from build123d import *

# Parameters (mm, degrees)
ESTRUSIONE_ESTRUSIONE5_DEPTH = 34
ESTRUSIONE_ESTRUSIONE6_DEPTH = 32
SCHIZZO9_R                   = 14.5
ESTRUSIONE_ESTRUSIONE7_DEPTH = 8
SCHIZZO10_R                  = 8
TAGLIO_ESTRUSIONE1_DEPTH     = 104.947101932
SCHIZZO11_R                  = 3
TAGLIO_ESTRUSIONE2_DEPTH     = 98.923439482
NERVATURA1_START             = -3
NERVATURA1_DEPTH             = 6
NERVATURA11_START            = -3
NERVATURA11_DEPTH            = 6


with BuildPart() as part:
    # Schizzo7 → Estrusione-Estrusione5 (new, symmetric)
    with BuildSketch(Plane(origin=(0, 0, 0), x_dir=(1, 0, 0), z_dir=(0, 1, 0))):
        Polygon((-57, 20), (-57, -20), (-47, -20), (-47, 10), (57, 10), (57, 50), (47, 50), (47, 20), align=None)
    extrude(amount=ESTRUSIONE_ESTRUSIONE5_DEPTH, both=True)

    # Schizzo8 → Estrusione-Estrusione6 (add)
    with BuildSketch(Plane.XY.offset(-10)):
        with BuildLine():
            Line((-27.5, 5.656854249), (-4.833333333, 13.670731103))
            ThreePointArc((-4.833333333, 13.670731103), (0, 14.5), (4.833333333, 13.670731103))
            Line((4.833333333, 13.670731103), (27.5, 5.656854249))
            ThreePointArc((27.5, 5.656854249), (31.5, 0), (27.5, -5.656854249))
            Line((27.5, -5.656854249), (4.833333333, -13.670731103))
            ThreePointArc((4.833333333, -13.670731103), (0, -14.5), (-4.833333333, -13.670731103))
            Line((-4.833333333, -13.670731103), (-27.5, -5.656854249))
            ThreePointArc((-27.5, -5.656854249), (-31.5, 0), (-27.5, 5.656854249))
        make_face()
    extrude(amount=ESTRUSIONE_ESTRUSIONE6_DEPTH)

    # Schizzo9 → Estrusione-Estrusione7 (add)
    with BuildSketch(Plane.XY.offset(22)):
        with Locations(Location((0, 0, 0), (0, 0, 109.471220634))):
            Circle(SCHIZZO9_R)
    extrude(amount=ESTRUSIONE_ESTRUSIONE7_DEPTH)

    # Schizzo10 → Taglio-Estrusione1 (cut, through all)
    with BuildSketch(Plane.XY.offset(30)):
        Circle(SCHIZZO10_R)
    extrude(amount=-TAGLIO_ESTRUSIONE1_DEPTH, mode=Mode.SUBTRACT)

    # Schizzo11 → Taglio-Estrusione2 (cut, through all)
    with BuildSketch(Plane.XY.offset(22)):
        with Locations((-25.1, 0)):
            Circle(SCHIZZO11_R)
        with Locations((25.9, 0)):
            Circle(SCHIZZO11_R)
    extrude(amount=-TAGLIO_ESTRUSIONE2_DEPTH, mode=Mode.SUBTRACT)

    # Nervatura1: read off the stored shape, not the designer's step
    # Nervatura1 outline → Nervatura1 (add)
    with BuildSketch(Plane(origin=(0, 0, 0), x_dir=(1, 0, 0), z_dir=(0, 1, 0)).offset(NERVATURA1_START)):
        Polygon((31.5, -22), (57, 10), (30.696152423, 10), (30.696152423, -22), align=None)
    extrude(amount=NERVATURA1_DEPTH)

    # Nervatura11: read off the stored shape, not the designer's step
    # Nervatura11 outline → Nervatura11 (add)
    with BuildSketch(Plane(origin=(0, 0, 0), x_dir=(1, 0, 0), z_dir=(0, 1, 0)).offset(NERVATURA11_START)):
        Polygon((-30.696152423, 10), (-47, 10), (-47, -20), (-31.5, -22), (-30.696152423, -22), align=None)
    extrude(amount=NERVATURA11_DEPTH)


solid = part.part
The listing builds one solid part. Answer for the finished solid, in the listing's coordinates (mm). A direction names the side the tool comes from. Give positions to 0.01 mm unless a question says otherwise; leave off trailing zeros. Write each loop counter-clockwise with the first axis right and the second up, starting at its lowest first coordinate (ties: lowest second). Pieces come first, ordered by that corner, then holes.
1) Section D-D (y = -27.5) is taken. Write down the section's boundary in (x, z).
2) A tool of negligible diameter and unlimited length cuts with its end or side. For faces 4 (the face through (-52, 0, 20)), 5 (the face through (-29.313, -4.633, 5.776)), 6 (the face through (-47, 19, 5)), 7 (the face through (16.325, -9.608, 5.776)), from which of +Z, -Z, +X, -X, +Y, -Y can it reach the whole face along a straight path? Write none if from no direction.
3) For a pull along X with two mould halves and no side action, classify faces 1 (the face through (-29.358, 4.595, 5.776)), 2 (the face through (47, 0, -35)), 3 (the face through (0, -34, -15)) as pulls with the +X half, pulls with the -X half, needs draft (parallel to the pull), parting line crosses it, or undercut.
4) Find the intervals of material crossed by L1, parallel to X at y = -3.5, z = 3; L2, parallel to Y at x = 0.5, z = 6; L3, parallel to Z at x = -44.5, y = -24, in increasing order.
5) Section A-A (y = 0) is taken. Write down the section's boundary in (x, z), and give its area (3 significant figures).
6) Section C-C (x = 0) is taken. Write down the section's boundary in (y, z), and give its area (3 significant figures).
7) Section B-B (z = -18) is taken. Write down the section's boundary in (x, y), and give its area (3 significant figures).
8) Given P1, Ø5, axis at x = -2.5, z = 2, coming from the +Y side; P2, Ø4, axis at y = 11.5, z = -38.5, coming from the -X side; P3, Ø5, axis at x = -51, y = -14, coming from the +Z side; P4, Ø5, axis at y = -1.5, z = -9.5, coming from the +X side, each flat-ended and moving along its own axis, determine where each tip first touches the part or whether it passes through.
Response:
1. outline: (-57, -20) - (47, -20) - (47, -50) - (57, -50) - (57, -10) - (-47, -10) - (-47, 20) - (-57, 20) - close
2. face 4: +Z, -X, +Y, -Y
2. face 5: +Z, -Y
2. face 6: +Z, +Y
2. face 7: +Z, +X, -Y
3. face 1: undercut
3. face 2: pulls with the -X half
3. face 3: needs draft
4. L1: x = -57 to -47, -30.37 to -7.19, 7.19 to 30.37
4. L2: y = -14.49 to -7.98, 7.98 to 14.49
4. L3: z = -20 to -10
5. outline: (-57, -20) - (-28.1, -20) - (-28.1, 22) - (-31.5, 22) - (-47, 20) - (-57, 20) - close; (-22.1, -20) - (-8, -20) - (-8, 30) - (-14.5, 30) - (-14.5, 22) - (-22.1, 22) - close; (8, -20) - (22.9, -20) - (22.9, 22) - (14.5, 22) - (14.5, 30) - (8, 30) - close; (28.9, -20) - (47, -20) - (47, -50) - (57, -50) - (57, -10) - (31.5, 22) - (28.9, 22) - close
5. area: 3,570 mm2
6. outline: (-34, -20) - (-8, -20) - (-8, 30) - (-14.5, 30) - (-14.5, -10) - (-34, -10) - close; (8, -20) - (34, -20) - (34, -10) - (14.5, -10) - (14.5, 30) - (8, 30) - close
6. area: 1,040 mm2
7. outline: (-57, -34) - (57, -34) - (57, 34) - (-57, 34) - close; hole circle Ø6 at (-25.1, 0); hole circle Ø16 at (0, 0); hole circle Ø6 at (25.9, 0)
7. area: 7,490 mm2
8. P1: stops at y = 14.5
8. P2: stops at x = 47
8. P3: stops at z = 20
8. P4: stops at x = 57
